from build123d import *

# Parameters (mm, degrees)
BOSS_EXTRUDE1_DEPTH     = 9
SKETCH2_R               = 1.625
CUT_EXTRUDE3_DEPTH      = 9
SKETCH8_W               = 9
SKETCH8_H               = 7
SKETCH8_R               = 1.625
BOSS_EXTRUDE2_DEPTH     = 6
CUT_EXTRUDE4_DEPTH      = 33
CUT_EXTRUDE4_DEPTH_BACK = 3
SKETCH9_R               = 2.875


with BuildPart() as part:
    # Sketch1 → Boss-Extrude1 (new body)
    # profile 1 of 3: a face of its own
    with BuildSketch(Plane.XY):
        Polygon((86.974134086, 0), (43.487067043, 43.487067043), (0, 0), align=None)
        Polygon((43.487067043, 35.001785669), (72.488852712, 6), (14.485281374, 6), align=None, mode=Mode.SUBTRACT)
    # profile 2 of 3: a face of its own
    with BuildSketch(Plane.XY):
        Polygon((34.487067043, 26.001785669), (29.749143655, 21.263862281), (36.866799529, 6), (43.487067043, 6), (36.957927158, 20.001785669), (43.487067043, 20.001785669), (43.487067043, 26.001785669), align=None)
    # profile 3 of 3: a face of its own
    with BuildSketch(Plane.XY):
        Polygon((50.016206928, 20.001785669), (43.487067043, 6), (50.107334557, 6), (57.224990431, 21.263862281), (52.487067043, 26.001785669), (43.487067043, 26.001785669), (43.487067043, 20.001785669), align=None)
    extrude(amount=BOSS_EXTRUDE1_DEPTH)

    # Sketch2 → Cut-Extrude3 (cut)
    with BuildSketch(Plane(origin=(0, 0, 0), x_dir=(0, 0, 1), z_dir=(-0.7071067811865438, 0.7071067811865513, 0))):
        with Locations(Location((4.5, 9, 0), (0, 0, 270))):
            Circle(SKETCH2_R)
    extrude(amount=-CUT_EXTRUDE3_DEPTH, mode=Mode.SUBTRACT)

    # Sketch8 → Boss-Extrude2 (add)
    with BuildSketch(Plane(origin=(0, 0, 0), x_dir=(0, 0, 1), z_dir=(-0.7071067811865438, 0.7071067811865513, 0))):
        with Locations((4.5, 65)):
            Rectangle(SKETCH8_W, SKETCH8_H)
        with Locations(Location((4.5, 65, 0), (0, 0, 270))):
            Circle(SKETCH8_R, mode=Mode.SUBTRACT)
    extrude(amount=-BOSS_EXTRUDE2_DEPTH)

    # Sketch9 → Cut-Extrude4 (cut, two sides: drawn at the far end of the back side and taken through both)
    with BuildSketch(Plane(origin=(4.242640687, -4.242640687, 0), x_dir=(0, 0, -1), z_dir=(0.7071067811865438, -0.7071067811865512, 0)).offset(-CUT_EXTRUDE4_DEPTH_BACK)):
        with Locations(Location((-4.5, 65, 0), (0, 0, 270))):
            Circle(SKETCH9_R)
        with Locations(Location((-4.5, 9, 0), (0, 0, 270))):
            Circle(SKETCH9_R)
    extrude(amount=CUT_EXTRUDE4_DEPTH + CUT_EXTRUDE4_DEPTH_BACK, mode=Mode.SUBTRACT)


solid = part.part
Read the model definition and answer for the solid it produces. Units are mm, in the model's axes. A direction names the side the tool comes from. Round coordinates to 2 decimals unless told otherwise and drop trailing zeros. Write each loop counter-clockwise with the first axis right and the second up, starting at its lowest first coordinate (ties: lowest second). Pieces come first, ordered by that corner, then holes.
Q1. Find section B-B on x = 65. Determine the outline of the cut face in (y, z).
Values:
outline: (0, 0) - (6, 0) - (6, 9) - (0, 9) - close; (13.49, 0) - (21.97, 0) - (21.97, 9) - (13.49, 9) - close
Q2. The mould has two halves that part along X. Classify faces 4 (the face through (38, 17, 9)), 5 (the face through (67.627, 19.348, 4.437)), 6 (the face through (40.27, 12.9, 4.44)), 7 (the face through (46.756, 42.514, 4.46)): released by +X, released by -X, zero draft, split by the parting line, or undercut.
Values:
face 4: zero draft
face 5: released by +X
face 6: undercut
face 7: undercut
Q3. A tool of negligible diameter and unlimited length cuts with its end or side. For faces 1 (the face through (22.01, 13.525, 4.437)), 2 (the face through (7.16, 2.92, 4.46)), 3 (the face through (38, 17, 0)), from which of +Z, -Z, +X, -X, +Y, -Y can it reach the whole face along a straight path? Write none if from no direction.
Values:
face 1: +Z, -Z
face 2: none
face 3: -Z, +X, -X, +Y, -Y
Q4. Straight lines are drawn through the part: line 1 (X direction, y = 12, z = 2.25); line 2 (X direction, y = 12.5, z = 1.5); line 3 (Y direction, x = 37.5, z = 8.75). For each, find the intervals that lie inside material, in ascending order.
Values:
line 1: x = 12 to 20.49, 34.07 to 40.69, 46.28 to 52.91, 66.49 to 74.97
line 2: x = 12.5 to 20.99, 33.84 to 40.46, 46.52 to 53.14, 65.99 to 74.47
line 3: y = 0 to 18.84, 20 to 26, 29.01 to 37.5
Q5. Find section A-A on y = 10. Determine the outline of the cut face in (x, z).
Values:
outline: (10, 0) - (18.49, 0) - (18.49, 9) - (10, 9) - close; (35, 0) - (41.62, 0) - (41.62, 9) - (35, 9) - close; (45.35, 0) - (51.97, 0) - (51.97, 9) - (45.35, 9) - close; (68.49, 0) - (76.97, 0) - (76.97, 9) - (68.49, 9) - close
Q6. Find section C-C on y = 33. Determine the outline of the cut face in (x, z).
Values:
outline: (33, 0) - (41.49, 0) - (41.49, 9) - (33, 9) - close; (45.49, 0) - (53.97, 0) - (53.97, 9) - (45.49, 9) - close
Q7. Find section D-D on x = 81.5. Determine the outline of the cut face in (y, z).
Values:
outline: (0, 0) - (5.47, 0) - (5.47, 9) - (0, 9) - close
Q8. Flat-ended cylindrical pins translate along their axes: P1, Ø2.5, axis at x = 28, z = 6, coming from the +Y side; P2, Ø3, axis at y = 11.5, z = 7, coming from the +X side; P3, Ø4, axis at x = 54, z = 7.5, coming from the +Y side. Find the tip coordinate at first contact, or state that the pin passes through.
Values:
P1: stops at y = 29.25
P2: stops at x = 76.97
P3: stops at y = 44.87
